The model under review builds one solid part; all positions refer to its coordinate system, in mm. Face numbers are marked on the shaded views. A direction names the side the tool comes from. Coordinates: 2 decimals unless noted, no trailing zeros. Loops run counter-clockwise (first coordinate to the right, second up) from the corner with the lowest first, then second, coordinate; pieces in that order, holes last. Notation, with made-up numbers: (-37.75, 65.5) - (11.25, 65.5) arc R15 ccw to (11.25, 76.5) - close; hole circle Ø2 at (83, 79.5). An arc over 180 degrees is marked (long way). One line per item, written item: value. Start each with the question number.
1. We need section B-B, the plane z = 16.5. Give the boundary of the cut face in (x, y), then the cut area to 3 significant figures.
2. Insertion check: P1, Ø5, axis at x = 14, y = -22, coming from the +Z side; P2, Ø6, axis at x = 16.5, z = 9, coming from the +Y side; P3, Ø8, axis at y = -18.5, z = 22.5, coming from the -X side; P4, Ø1.5, axis at x = -20.5, z = 15.5, coming from the +Y side. Each pin has a flat end and moves straight along its axis. Give the tip position at first contact, or say it passes through.
3. We need section A-A, the plane x = 16.5. Give the boundary of the cut face in (y, z).
4. We need section C-C, the plane y = 16.5. Give the boundary of the cut face in (x, z), then the cut area to 3 significant figures.
5. Mouldability with a two-part tool opening along X and no side actions: class the marked faces 1, 2 and 3 as +X half, -X half, draft (parallel to the pull), parting line (faces both ways), or undercut.
6. We need section D-D, the plane y = -2. Give the boundary of the cut face in (x, z), then the cut area to 3 significant figures.
7. For the marked faces 4 and 5, list the 3-axis set-ups (+Z, -Z, +X, -X, +Y, -Y) from which the entire face can be reached by the end or side of a thin tool; tool diameter is ignored.
8. To check wall thickness, follow line 1 (X direction, y = -29.55, z = 16.5); line 2 (Y direction, x = -15.5, z = 1.75); line 3 (Y direction, x = -3.5, z = 3). State the ranges of each line that lie inside material, in increasing order.
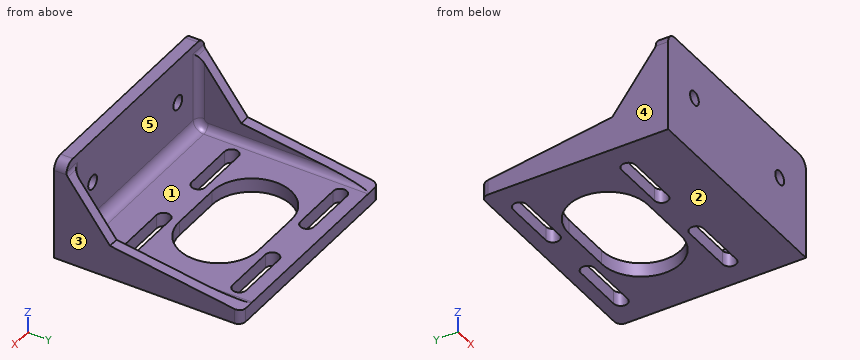
from build123d import *

# Parameters (mm, degrees)
SKETCH_1_W          = 62.922128066
SKETCH_1_H          = 53.34190314
EXTRUDE_1_DEPTH     = 4
SKETCH_2_W          = 62.922128066
SKETCH_2_H          = 3.5
EXTRUDE_2_DEPTH     = 25
CUT_EXTRUDE_1_REACH = 67.689
SKETCH_3_R          = 2
FILLET_1_R          = 3
EXTRUDE_3_DEPTH     = 3
EXTRUDE_4_DEPTH     = 3
FILLET_2_R          = 2


with BuildPart() as part:
    # Эскиз1 → Бобышка-Вытянуть1 (new body)
    with BuildSketch(Plane.XY):
        with Locations((0, -5.32904843)):
            Rectangle(SKETCH_1_W, SKETCH_1_H)
        with BuildLine():
            Line((-7.5, 11.25), (7.5, 11.25))
            ThreePointArc((7.5, 11.25), (18.75, 0), (7.5, -11.25))
            Line((7.5, -11.25), (-7.5, -11.25))
            ThreePointArc((-7.5, -11.25), (-18.75, 0), (-7.5, 11.25))
        make_face(mode=Mode.SUBTRACT)
        with BuildLine():
            Line((-23, 17.468671613), (-8, 17.468671613))
            ThreePointArc((-8, 17.468671613), (-6.031328387, 15.5), (-8, 13.531328387))
            Line((-8, 13.531328387), (-23, 13.531328387))
            ThreePointArc((-23, 13.531328387), (-24.968671613, 15.5), (-23, 17.468671613))
        make_face(mode=Mode.SUBTRACT)
        with BuildLine():
            Line((8.035969411, 17.506216751), (23.035969411, 17.506216751))
            ThreePointArc((23.035969411, 17.506216751), (25.004641024, 15.537545138), (23.035969411, 13.568873525))
            Line((23.035969411, 13.568873525), (8.035969411, 13.568873525))
            ThreePointArc((8.035969411, 13.568873525), (6.067297798, 15.537545138), (8.035969411, 17.506216751))
        make_face(mode=Mode.SUBTRACT)
        with BuildLine():
            Line((-23.022315975, -13.49101169), (-8.022315975, -13.49101169))
            ThreePointArc((-8.022315975, -13.49101169), (-6.053644362, -15.459683303), (-8.022315975, -17.428354916))
            Line((-8.022315975, -17.428354916), (-23.022315975, -17.428354916))
            ThreePointArc((-23.022315975, -17.428354916), (-24.990987588, -15.459683303), (-23.022315975, -13.49101169))
        make_face(mode=Mode.SUBTRACT)
        with BuildLine():
            Line((8.028946211, -13.4897295), (23.028946211, -13.4897295))
            ThreePointArc((23.028946211, -13.4897295), (24.997617824, -15.458401113), (23.028946211, -17.427072726))
            Line((23.028946211, -17.427072726), (8.028946211, -17.427072726))
            ThreePointArc((8.028946211, -17.427072726), (6.060274598, -15.458401113), (8.028946211, -13.4897295))
        make_face(mode=Mode.SUBTRACT)
    extrude(amount=EXTRUDE_1_DEPTH)

    # Эскиз2 → Бобышка-Вытянуть2 (add)
    with BuildSketch(Plane.XY.offset(4)):
        with Locations((0, -30.25)):
            Rectangle(SKETCH_2_W, SKETCH_2_H)
    extrude(amount=EXTRUDE_2_DEPTH)

    # Эскиз3 → Вырез-Вытянуть1 (cut, up to next)
    with BuildSketch(Plane(origin=(0, -28.5, 0), x_dir=(1, 0, 0), z_dir=(0, 1, 0)), mode=Mode.PRIVATE) as cut_extrude_1_sk1:
        with Locations(Location((-19.461064033, -16.5, 0), (0, 0, 270))):
            Circle(SKETCH_3_R)
    cut_extrude_1_tool1 = extrude(cut_extrude_1_sk1.sketch, amount=-CUT_EXTRUDE_1_REACH, mode=Mode.PRIVATE) & part.part
    # Эскиз3 → Вырез-Вытянуть1 (cut, up to next)
    with BuildSketch(Plane(origin=(0, -28.5, 0), x_dir=(1, 0, 0), z_dir=(0, 1, 0)), mode=Mode.PRIVATE) as cut_extrude_1_sk2:
        with Locations(Location((19.461064033, -16.5, 0), (0, 0, 270))):
            Circle(SKETCH_3_R)
    cut_extrude_1_tool2 = extrude(cut_extrude_1_sk2.sketch, amount=-CUT_EXTRUDE_1_REACH, mode=Mode.PRIVATE) & part.part
    add(cut_extrude_1_tool1.solids().sort_by_distance((-19.461064, -28.5, 16.5))[0], mode=Mode.SUBTRACT)
    add(cut_extrude_1_tool2.solids().sort_by_distance((19.461064, -28.5, 16.5))[0], mode=Mode.SUBTRACT)

    # Скругление1
    fillet_1_edges = [part.edges().sort_by_distance(p)[0] for p in [
        (0, -28.5, 4),
        (-31.461064033, -30.25, 29),
        (31.461064033, -30.25, 29),
    ]]
    fillet(fillet_1_edges, radius=FILLET_1_R)

    # Эскиз4 → Бобышка-Вытянуть3 (add)
    with BuildSketch(Plane(origin=(31.461064033, 0, 0), x_dir=(0, 0, -1), z_dir=(1, 0, 0))):
        Polygon((-26, -28.5), (-4, -28.5), (-4, 21.34190314), (-9.595875894, -16.066108025), align=None)
    extrude(amount=-EXTRUDE_3_DEPTH)

    # Эскиз5 → Бобышка-Вытянуть4 (add)
    with BuildSketch(Plane.ZY.offset(31.461064033)):
        Polygon((26, -28.5), (4, -28.5), (4, 21.34190314), (9.595875894, -16.066108025), align=None)
    extrude(amount=-EXTRUDE_4_DEPTH)

    # Скругление2
    fillet_2_edges = [part.edges().sort_by_distance(p)[0] for p in [
        (28.461064033, -27.621320344, 4.878679656),
        (28.461064033, -2.07904843, 4),
        (29.961064033, -28.5, 26),
        (28.461064033, -28.5, 16.5),
        (-28.461064033, -27.621320344, 4.878679656),
        (-28.461064033, -2.07904843, 4),
        (-28.461064033, -28.5, 16.5),
        (-29.961064033, -28.5, 26),
        (-31.461064033, 21.34190314, 2),
        (31.461064033, 21.34190314, 2),
    ]]
    fillet(fillet_2_edges, radius=FILLET_2_R)


solid = part.part
Findings below:
1. outline: (-31.46, -32) - (-21.46, -32) - (-21.46, -28.5) - (-26.46, -28.5) arc R2 cw to (-28.46, -26.5) - (-28.46, -21.3) - (-31.46, -21.3) - close; (-17.46, -32) - (17.46, -32) - (17.46, -28.5) - (-17.46, -28.5) - close; (21.46, -32) - (31.46, -32) - (31.46, -21.3) - (28.46, -21.3) - (28.46, -26.5) arc R2 cw to (26.46, -28.5) - (21.46, -28.5) - close
1. area: 237 mm2
2. P1: z = 4
2. P2: y = -28.33
2. P3: through
2. P4: y = -28.5
3. outline: (-32, 0) - (-17.43, 0) - (-17.43, 4) - (-25.5, 4) arc R3 cw to (-28.5, 7) - (-28.5, 29) - (-32, 29) - close; (-13.49, 0) - (-6.75, 0) - (-6.75, 4) - (-13.49, 4) - close; (6.75, 0) - (13.57, 0) - (13.57, 4) - (6.75, 4) - close; (17.51, 0) - (21.34, 0) - (21.34, 4) - (17.51, 4) - close
4. outline: (-31.46, 0) - (-24.7, 0) - (-24.7, 4) - (-26.46, 4) arc R2 cw to (-28, 4.72) - (-31.46, 4.72) - close; (-6.3, 0) - (6.32, 0) - (6.32, 4) - (-6.3, 4) - close; (24.75, 0) - (31.46, 0) - (31.46, 4.72) - (28, 4.72) arc R2 cw to (26.46, 4) - (24.75, 4) - close
4. area: 110 mm2
5. face 1: undercut
5. face 2: draft
5. face 3: +X half
6. outline: (-31.46, 0) - (-18.57, 0) - (-18.57, 4) - (-26.46, 4) arc R2 cw to (-28.46, 6) - (-28.46, 7.49) - (-31.46, 7.49) - close; (18.57, 0) - (31.46, 0) - (31.46, 7.49) - (28.46, 7.49) - (28.46, 6) arc R2 cw to (26.46, 4) - (18.57, 4) - close
6. area: 126 mm2
7. face 4: +Z, -Z, -X, +Y, -Y
7. face 5: +Z, +Y
8. line 1: -31.46 to -21.46, -17.46 to 17.46, 21.46 to 31.46
8. line 2: -32 to -17.43, -13.49 to -7.91, 7.91 to 13.53, 17.47 to 21.34
8. line 3: -32 to -11.25, 11.25 to 21.34
